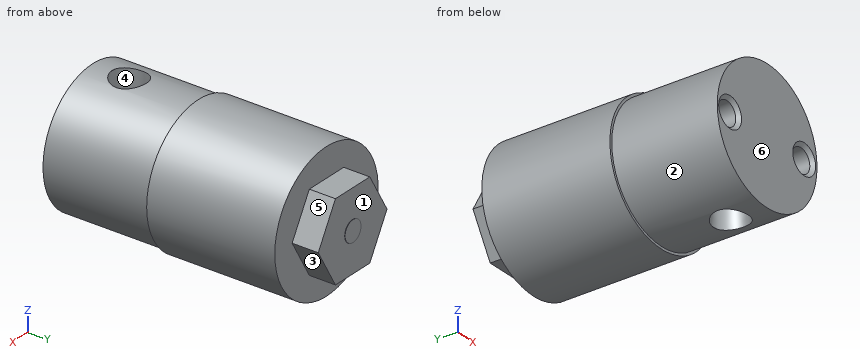
from build123d import *

# Parameters (mm, degrees)
ESQUISSE1_R               = 12.56
BOSS_EXTRU_1_DEPTH        = 20.19
ESQUISSE13_R              = 2
BOSS_EXTRU_2_DEPTH        = 29.59
ESQUISSE14_R              = 13.03
BOSS_EXTRU_3_DEPTH        = 24.51
BOSS_EXTRU_4_DEPTH        = 5
D_GAGEMENT_81_D           = 4.4958
D_GAGEMENT_81_DEPTH       = 8.649325414
D_GAGEMENT_81_CSINK_D     = 5.7658
D_GAGEMENT_81_CSINK_ANGLE = 90
D_GAGEMENT_81_TIP         = 1.350674586


with BuildPart() as part:
    # Esquisse1 → Boss.-Extru.1 (new body)
    with BuildSketch(Plane(origin=(0, 0, 0), x_dir=(1, 0, 0), z_dir=(0, 1, 0))):
        Circle(ESQUISSE1_R)
    extrude(amount=BOSS_EXTRU_1_DEPTH)

    # Esquisse9 → Trou taraudé 1/8 Rc1 (revolve, cut)
    with BuildSketch(Plane(origin=(0, 6.96, 12.56), x_dir=(0, -1, 0), z_dir=(1, 0, 0))):
        Polygon((0, 0), (0, 10.873399445), (3.95, 8.5), (3.95, 7.4), (3.05277742, 7.4), (3.283, 0.025), (3.308, 0), align=None)
    revolve(axis=Axis((0, 6.96, 18.91), (0, 0, -1)), mode=Mode.SUBTRACT)

    # Esquisse12 → Trou taraudé 1/8 Rc2 (revolve, cut)
    with BuildSketch(Plane(origin=(0, 6.949571946, -12.56), x_dir=(0, 1, 0), z_dir=(1, 0, 0))):
        Polygon((0, 0), (0, 10.873399445), (3.95, 8.5), (3.95, 7.4), (3.05277742, 7.4), (3.283, 0.025), (3.308, 0), align=None)
    revolve(axis=Axis((0, 6.949571946, -18.91), (0, 0, 1)), mode=Mode.SUBTRACT)

    # Esquisse13 → Boss.-Extru.2 (add)
    with BuildSketch(Plane(origin=(0, 20.19, 0), x_dir=(1, 0, 0), z_dir=(0, 1, 0))):
        Circle(ESQUISSE13_R)
    extrude(amount=BOSS_EXTRU_2_DEPTH)

    # Esquisse14 → Boss.-Extru.3 (add)
    with BuildSketch(Plane(origin=(0, 20.19, 0), x_dir=(1, 0, 0), z_dir=(0, 1, 0))):
        Circle(ESQUISSE14_R)
    extrude(amount=BOSS_EXTRU_3_DEPTH)

    # Esquisse16 → Boss.-Extru.4 (add)
    with BuildSketch(Plane(origin=(0, 44.7, 0), x_dir=(1, 0, 0), z_dir=(0, 1, 0))):
        Polygon((8.660254038, 0), (4.330127019, 7.5), (-4.330127019, 7.5), (-8.660254038, 0), (-4.330127019, -7.5), (4.330127019, -7.5), align=None)
    extrude(amount=BOSS_EXTRU_4_DEPTH)

    # Dégagement #81
    with Locations(Plane(origin=(-9.335, 0, 0), x_dir=(0, 0, -1), z_dir=(0, -1, 0))):
        with Locations((0, 0), (0, 18.67)):
            CounterSinkHole(D_GAGEMENT_81_D / 2, D_GAGEMENT_81_CSINK_D / 2, depth=D_GAGEMENT_81_DEPTH, counter_sink_angle=D_GAGEMENT_81_CSINK_ANGLE)
            with Locations((0, 0, -(D_GAGEMENT_81_DEPTH + D_GAGEMENT_81_TIP / 2))):  # 118° drill point
                Cone(0, D_GAGEMENT_81_D / 2, D_GAGEMENT_81_TIP, mode=Mode.SUBTRACT)


solid = part.part
Work out the finished part from the listing and answer in its coordinate system (mm). Face numbers are marked on the shaded views. A direction names the side the tool comes from. Give positions to 0.01 mm unless a question says otherwise; leave off trailing zeros. Loops run counter-clockwise (first coordinate to the right, second up) from the corner with the lowest first, then second, coordinate; pieces in that order, holes last. Notation, with made-up numbers: (35, -2.75) -> (81, -2.75) arc R21 cw to (81, 31.25) -> close; hole circle Ø11 at (78, 74). An arc over 180 degrees is marked (long way). Use a Markdown table: item, result. Add a question column.
1) Which of the six approach directions +Z, -Z, +X, -X, +Y, -Y give full straight-line access (tool end or side, diameter ignored) to the marked faces 1, 2 and 3?
2) For a pull along X with two mould halves and no side action, classify the marked faces 4, 5 and 6 as +X half, -X half, draft (parallel to the pull), parting line (faces both ways), or undercut.
3) The part is cut by section B-B, the plane y = 38. Determine the outline of the cut face in (x, z).
4) Each of these flat-tipped pins is pushed along its axis until it touches: P1, Ø5, axis at x = 8, y = 37, coming from the +Z side; P2, Ø8.5, axis at x = -0.5, y = 6, coming from the +Z side; P3, Ø4.5, axis at x = 0, y = 6.96, coming from the +Z side. Where does it stop, or does it pass through?
5) The part is cut by section A-A, the plane z = -6.5. Determine the outline of the cut face in (x, y), plus the area to 3 significant figures.
6) Consider line 1 along X through (y, z) = (4.5, 0); line 2 along Y through (x, z) = (0, -4.35); line 3 along Z through (x, y) = (0.5, 41). Determine where each line is inside the solid, lowest interval first.
Reported:
| question | item | result |
|---|---|---|
| 1 | face 1 | +Y |
| 1 | face 2 | -Y |
| 1 | face 3 | -Z, +X, +Y |
| 2 | face 4 | undercut |
| 2 | face 5 | +X half |
| 2 | face 6 | draft |
| 3 | outline | circle Ø26.06 at (0, 0) |
| 4 | P1 | stops at z = 11.81 |
| 4 | P2 | stops at z = 12.56 |
| 4 | P3 | stops at z = 3.04 |
| 5 | outline | (-11.29, 20.19) -> (-10.75, 20.19) -> (-10.75, 0) -> (10.75, 0) -> (10.75, 20.19) -> (11.29, 20.19) -> (11.29, 44.7) -> (4.91, 44.7) -> (4.91, 49.7) -> (-4.91, 49.7) -> (-4.91, 44.7) -> (-11.29, 44.7) -> close; hole circle Ø6.19 at (0, 6.95) |
| 5 | area | 1,010 mm^2 |
| 6 | line 1 | x = -12.56 to -11.58, -7.09 to 7.09, 11.58 to 12.56 |
| 6 | line 2 | y = 0 to 3, 10.9 to 49.7 |
| 6 | line 3 | z = -13.02 to 13.02 |
